Autodesk Inventor part; units mm, degrees
ref_plane "YZ Plane" through (0, 0, 0) normal (1, 0, 0) x (0, 1, 0)
ref_plane "XZ Plane" through (0, 0, 0) normal (0, 1, 0) x (-1, 0, 0)
ref_plane "XY Plane" through (0, 0, 0) normal (0, 0, 1) x (1, 0, 0)
sketch "Sketch1" plane through (0, 0, 0) normal (1, 0, 0) x (0, 1, 0)
  line L0 (0, 0) -> (10, 0)
  line L1 (10, 0) -> (0, -20)
  line L2 (0, -20) -> (0, 0)
  dimension "d0" = 20
  dimension "d1" = 10
extrude "Extrusion1" add sketch "Sketch1" along normal blind 35
sketch "Sketch7" plane through (0, 0, -20) normal (0, -1, 0) x (1, 0, 0)
  line L0 (35, 20) -> (35, 0)
  line L1 (0, 0) -> (0, 20)
  line L2 (35, 0) -> (0, 0)
  line L3 (0, 0) -> (0, 5)
  line L4 (0, 5) -> (35, 5)
  line L5 (35, 5) -> (35, 0)
  dimension "d17" = 5
extrude "Extrusion7" add sketch "Sketch7" along normal blind 11
sketch "Sketch8" plane through (0, 0, -15) normal (0, 0, 1) x (1, 0, 0)
  line L0 (35, -11) -> (0, -11)
  line L1 (0, -11) -> (0, -5.5)
  line L2 (0, -5.5) -> (35, -5.5)
  line L3 (35, -5.5) -> (35, -11)
  point P0 (0, 0)
  dimension "d20" = 5.5
  dimension "d26" = 35
extrude "Extrusion8" add sketch "Sketch8" along normal blind 15
sketch "Sketch9" plane through (0, -11, -20) normal (0, -1, 0) x (1, 0, 0)
  line L0 (0, 5) -> (0, 20)
  line L1 (35, 0) -> (0, 0)
  line L2 (0, 0) -> (0, 5)
  line L3 (0, 5) -> (35, 5)
  line L4 (35, 5) -> (35, 0)
  dimension "d23" = 5
extrude "Extrusion9" add sketch "Sketch9" along normal blind 20
sketch "Sketch10" plane through (35, 0, 0) normal (1, 0, 0) x (0, 0, -1)
  line L0 (15, 0) -> (0, 0)
  line L1 (0, 0) -> (-10, 0)
  line L2 (0, -11) -> (-10, -11)
  line L3 (-10, -11) -> (-10, -5.5)
  line L4 (-10, -5.5) -> (0, -5.5)
  line L5 (0, -5.5) -> (0, -11)
  line L6 (0, 10) -> (20, 0)
  line L7 (0, 10) -> (-10, 15)
  line L8 (20, 0) -> (0, 10)
  line L9 (-10, 0) -> (-10, 15)
  line L10 (0, 0) -> (0, 10)
  line L11 (0, 0) -> (0, 10)
  dimension "d27" = 10
  dimension "d30" = 10
extrude "Extrusion10" add sketch "Sketch10" against normal blind 25
properties part number "Ooze_Ramp_Top"
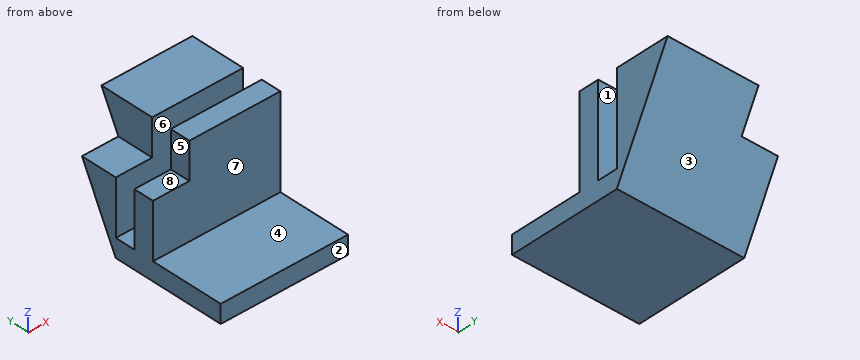
Part model, mm, in its own coordinate system. Face numbers are marked on the shaded views. A direction names the side the tool comes from. Give positions to 0.01 mm unless a question says otherwise; leave off trailing zeros. Write each loop counter-clockwise with the first axis right and the second up, starting at its lowest first coordinate (ties: lowest second). Pieces come first, ordered by that corner, then holes.
1) Cut at A-A on z = -1.5. Write the cut outline in (x, y), then the cut area to 3 significant figures.
Resolved:
outline: (0, -11) - (35, -11) - (35, -5.5) - (0, -5.5) - close; (0, 0) - (35, 0) - (35, 9.25) - (0, 9.25) - close
area: 516 mm2
2) Which spindle directions (+Z, -Z, +X, -X, +Y, -Y) get a long thin tool onto all of the face, cutting with end or side? Do the marked faces 1, 2, 3, 4 and 5. Say none if no direction does.
Resolved:
face 1: +Z, +X, -X
face 2: +Z, -Z, +X, -X, -Y
face 3: -Z, +X, -X, +Y
face 4: +Z, +X, -X, -Y
face 5: +Z, -X, +Y, -Y
3) Cut at C-C on y = 5.5. Write the cut outline in (x, z), then the cut area to 3 significant figures.
Resolved:
outline: (0, -9) - (35, -9) - (35, 10) - (10, 10) - (10, 0) - (0, 0) - close
area: 565 mm2
4) Probe L1, parallel to Z at x = 5, y = -25; L2, parallel to Z at x = 5, y = 2.5; L3, parallel to X at y = 7, z = 8.75. List the from-to ranges inside material, lowest first.
Resolved:
L1: z = -20 to -15
L2: z = -15 to 0
L3: x = 10 to 35
5) Cut at B-B on x = 17. Write the cut outline in (y, z), then the cut area to 4 significant figures.
Resolved:
outline: (-31, -20) - (0, -20) - (15, 10) - (0, 10) - (0, -15) - (-5.5, -15) - (-5.5, 10) - (-11, 10) - (-11, -15) - (-31, -15) - close
area: 517.5 mm2
6) Two-plate mould, pull along Y, no slides. Class the marked faces 6, 7 and 8: released by +Y, released by -Y, zero draft, split by the parting line, or undercut.
Resolved:
face 6: undercut
face 7: released by -Y
face 8: zero draft
7) Cut at D-D on z = 7.75. Write the cut outline in (x, y) (3 decimals).
Resolved:
outline: (10, -11) - (35, -11) - (35, -5.5) - (10, -5.5) - close; (10, 0) - (35, 0) - (35, 13.875) - (10, 13.875) - close
8) Pin check, flat tips, straight feed: pin 1 (1.6 mm diameter, centred on y = -9, z = 5.5, fed in from -X); pin 2 (16 mm diameter, centred on x = 26, y = -23, fed in from +Z); pin 3 (7.5 mm diameter, centred on x = 10.5, z = -1, fed in from +Y) (3 decimals). Stop position of each tip, or through.
Resolved:
pin 1: stops at x = 10
pin 2: stops at z = -15
pin 3: stops at y = 11.375
